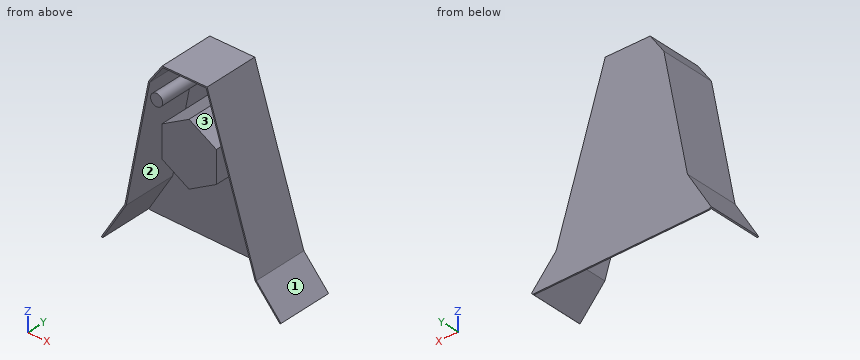
from build123d import *

# Parameters (mm, degrees)
SKETCH_2_R        = 9
EXTRUDE_1_DEPTH   = 80
EXTRUDE_1_2_DEPTH = 80
EXTRUDE_1_3_DEPTH = 80
EXTRUDE_2_DEPTH   = 2


with BuildPart() as part:
    # Sketch 2 → Extrude 1 (new body)
    with BuildSketch(Plane(origin=(0, 0, 0), x_dir=(1, 0, 0), z_dir=(0, 1, 0))):
        with Locations((-100.00360092, 94.257346069)):
            Circle(SKETCH_2_R)
    extrude(amount=EXTRUDE_1_DEPTH)



with BuildPart() as body_2:
    # Sketch 2 → Extrude 1 2 (new body)
    with BuildSketch(Plane(origin=(0, 0, 0), x_dir=(1, 0, 0), z_dir=(0, 1, 0))):
        Polygon((-180.407965552, 313.211742037), (-145.137395052, 254.599587646), (-110.045954215, 74.705720884), (-90.558125094, 46.975459978), (-26.188648694, 46.975459978), (46.650236815, 274.975459978), (83.703115643, 317.123903245), (85.205209719, 315.803405844), (48.428218628, 273.968790786), (-24.728005079, 44.975459978), (-91.597082511, 44.975459978), (-111.927353435, 73.904475802), (-147.032877617, 253.870539869), (-182.121617812, 312.180531131), align=None)
    extrude(amount=EXTRUDE_1_2_DEPTH)


with BuildPart() as body_3:
    # Sketch 2 → Extrude 1 3 (new body)
    with BuildSketch(Plane(origin=(0, 0, 0), x_dir=(1, 0, 0), z_dir=(0, 1, 0))):
        Polygon((-51.670033073, 193.433505049), (-92.281031996, 169.986733889), (-92.281031996, 123.093191569), (-51.670033073, 99.646420409), (-11.059034151, 123.093191569), (-11.059034151, 169.986733889), align=None)
    extrude(amount=EXTRUDE_1_3_DEPTH)


with BuildPart() as part_1:
    add(part.part)

    add(body_2.part)  # Extrude 2 merges body 2

    add(body_3.part)  # Extrude 2 merges body 3
    # Sketch 3 → Extrude 2 (add)
    with BuildSketch(Plane(origin=(0, 80, 0), x_dir=(1, 0, 0), z_dir=(0, 1, 0))):
        Polygon((-178.746676914, 314.325348818), (81.764058494, 317.613859747), (83.703115643, 317.123903245), (85.205209719, 315.803405844), (48.428218628, 273.968790786), (-24.728005079, 44.975459978), (-91.597082511, 44.975459978), (-111.927353435, 73.904475802), (-147.032877617, 253.870539869), (-182.121617812, 312.180531131), (-180.407965552, 313.211742037), align=None)
    extrude(amount=EXTRUDE_2_DEPTH)


solid = part_1.part
The model under review builds one solid part; all positions refer to its coordinate system, in mm. Face numbers are marked on the shaded views. A direction names the side the tool comes from. Round coordinates to 2 decimals unless told otherwise and drop trailing zeros. Write each loop counter-clockwise with the first axis right and the second up, starting at its lowest first coordinate (ties: lowest second). Pieces come first, ordered by that corner, then holes. Notation, with made-up numbers: M 84.5,-15 L 109.5,-15 A19 cw 109.5,1 Z; hole C 46,-38.75 d7. An arc over 180 degrees is marked long. Use a Markdown table: item, result. Add a question column.
Q1. We need section A-A, the plane y = 31. State the section outline as (x, z) points, plus the area to 3 significant figures.
Q2. Insertion check: pin 1 (2 mm diameter, centred on y = 36, z = -192, fed in from -X); pin 2 (1 mm diameter, centred on x = 49.5, y = 57.5, fed in from -Z); pin 3 (4 mm diameter, centred on y = 64, z = -246.5, fed in from -X). Each pin has a flat end and moves straight along its axis. Give the tip position at first contact, or say it passes through.
Q3. We need section B-B, the plane z = -180. State the section outline as (x, y) points, plus the area to 3 significant figures.
Q4. We need section C-C, the plane x = -58. State the section outline as (y, z) points.
Q5. Machinability: for the marked faces 1, 2 and 3, which of the approach directions +Z, -Z, +X, -X, +Y, -Y give a long, thin tool a straight path to every point of the face, cutting with its end or side? Answer none if there is none.
Q6. We need section D-D, the plane z = -127. State the section outline as (x, y) points, plus the area to 3 significant figures.
Q7. To check wall thickness, follow line 1 (X direction, y = 49, z = -110); line 2 (X direction, y = 27, z = -137.5); line 3 (X direction, y = 52.5, z = -240.5). State the ranges of each line that lie inside material, in increasing order.
Findings below:
| question | item | result |
|---|---|---|
| 1 | outline | M -182.12,-312.18 L -180.41,-313.21 L -145.14,-254.6 L -110.05,-74.71 L -90.56,-46.98 L -26.19,-46.98 L 46.65,-274.98 L 83.7,-317.12 L 85.21,-315.8 L 48.43,-273.97 L -24.73,-44.98 L -91.6,-44.98 L -111.93,-73.9 L -147.03,-253.87 Z; C -100,-94.26 d18; M -92.28,-169.99 L -51.67,-193.43 L -11.06,-169.99 L -11.06,-123.09 L -51.67,-99.65 L -92.28,-123.09 Z |
| 1 | area | 7,260 mm² |
| 2 | pin 1 | stops at x = -135.16 |
| 2 | pin 2 | stops at z = -278.79 |
| 2 | pin 3 | stops at x = -145.99 |
| 3 | outline | M -132.62,0 L -130.59,0 L -130.59,80 L -74.94,80 L -74.94,0 L -28.4,0 L -28.4,80 L 16.31,80 L 16.31,0 L 18.41,0 L 18.41,82 L -132.62,82 Z |
| 3 | area | 4,360 mm² |
| 4 | outline | M 0,-189.78 L 80,-189.78 L 80,-315.85 L 82,-315.85 L 82,-44.98 L 0,-44.98 L 0,-46.98 L 80,-46.98 L 80,-103.3 L 0,-103.3 Z |
| 5 | face 1 | +Z, +X, +Y, -Y |
| 5 | face 2 | -Z, -Y |
| 5 | face 3 | -Y |
| 6 | outline | M -122.28,0 L -120.25,0 L -120.25,80 L -92.28,80 L -92.28,0 L -11.06,0 L -11.06,80 L -0.62,80 L -0.62,0 L 1.48,0 L 1.48,82 L -122.28,82 Z |
| 6 | area | 7,080 mm² |
| 7 | line 1 | x = -118.97 to -116.93, -69.6 to -33.74, -6.05 to -3.95 |
| 7 | line 2 | x = -124.33 to -122.3, -92.28 to -11.06, 2.73 to 4.83 |
| 7 | line 3 | x = -144.42 to -142.39, 35.64 to 37.74 |
